from build123d import *

# Parameters (mm, degrees)
SKETCH1_R                   = 3.302
SKETCH1_R_2                 = 2.54
BOSS_EXTRUDE1_DEPTH         = 3.937
BODY_MOVE_COPY1_OUTLINE_R   = 2.54
BODY_MOVE_COPY1_DEPTH       = 3.937
BODY_MOVE_COPY1_2_OUTLINE_R = 2.54
BODY_MOVE_COPY1_2_DEPTH     = 3.937
SKETCH2_R                   = 3.302
CUT_EXTRUDE1_DEPTH          = 0.635


# Read off the part's stored shape, not the designer's step: Body-Move/Copy1
with BuildPart() as part:
    # Sketch1 → Boss-Extrude1 (new body)
    # profile 1 of 4: a face of its own
    with BuildSketch(Plane.XY):
        with BuildLine():
            Line((3.937, -3.81), (7.874, -3.81))
            ThreePointArc((7.874, -3.81), (11.684, 0), (7.874, 3.81))
            Line((7.874, 3.81), (3.937, 3.81))
            Line((3.937, 3.81), (3.937, 3.302))
            Line((3.937, 3.302), (4.92278669, 3.302))
            ThreePointArc((4.92278669, 3.302), (5.389414486, 2.994804631), (5.291688354, 2.44475))
            ThreePointArc((5.291688354, 2.44475), (4.318, 0), (5.291688354, -2.44475))
            ThreePointArc((5.291688354, -2.44475), (5.389414486, -2.994804631), (4.92278669, -3.302))
            Line((4.92278669, -3.302), (3.937, -3.302))
            Line((3.937, -3.302), (3.937, -3.81))
        make_face()
        with Locations((7.874, 0)):
            Circle(SKETCH1_R, mode=Mode.SUBTRACT)
    # profile 2 of 4: a face of its own
    with BuildSketch(Plane.XY):
        with Locations((7.874, 0)):
            Circle(SKETCH1_R)
        with Locations((7.874, 0)):
            Circle(SKETCH1_R_2, mode=Mode.SUBTRACT)
    # profile 3 of 4: a face of its own
    with BuildSketch(Plane.XY):
        with BuildLine():
            Line((-7.874, -3.81), (-3.937, -3.81))
            Line((-3.937, -3.81), (-3.937, -3.302))
            Line((-3.937, -3.302), (-4.92278669, -3.302))
            ThreePointArc((-4.92278669, -3.302), (-5.389414486, -2.994804631), (-5.291688354, -2.44475))
            ThreePointArc((-5.291688354, -2.44475), (-4.318, 0), (-5.291688354, 2.44475))
            ThreePointArc((-5.291688354, 2.44475), (-5.389414486, 2.994804631), (-4.92278669, 3.302))
            Line((-4.92278669, 3.302), (-3.937, 3.302))
            Line((-3.937, 3.302), (-3.937, 3.81))
            Line((-3.937, 3.81), (-7.874, 3.81))
            ThreePointArc((-7.874, 3.81), (-11.684, 0), (-7.874, -3.81))
        make_face()
        with Locations((-7.874, 0)):
            Circle(SKETCH1_R, mode=Mode.SUBTRACT)
    # profile 4 of 4: a face of its own
    with BuildSketch(Plane.XY):
        with Locations((-7.874, 0)):
            Circle(SKETCH1_R)
        with Locations((-7.874, 0)):
            Circle(SKETCH1_R_2, mode=Mode.SUBTRACT)
    extrude(amount=BOSS_EXTRUDE1_DEPTH)

    # Body-Move/Copy1 outline → Body-Move/Copy1 (cut)
    with BuildSketch(Plane.XY):
        with BuildLine():
            ThreePointArc((-7.874, 3.81), (-11.684, 0), (-7.874, -3.81))
            Line((-7.874, -3.81), (-3.937, -3.81))
            Line((-3.937, -3.81), (-3.937, -3.302))
            Line((-3.937, -3.302), (-4.92278669, -3.302))
            ThreePointArc((-4.92278669, -3.302), (-5.389414486, -2.994804631), (-5.291688354, -2.44475))
            ThreePointArc((-5.291688354, -2.44475), (-4.318, 0), (-5.291688354, 2.44475))
            ThreePointArc((-5.291688354, 2.44475), (-5.389414486, 2.994804631), (-4.92278669, 3.302))
            Line((-4.92278669, 3.302), (-3.937, 3.302))
            Line((-3.937, 3.302), (-3.937, 3.81))
            Line((-3.937, 3.81), (-7.874, 3.81))
        make_face()
        with Locations((-7.874, 0)):
            Circle(BODY_MOVE_COPY1_OUTLINE_R, mode=Mode.SUBTRACT)
    extrude(amount=BODY_MOVE_COPY1_DEPTH, mode=Mode.SUBTRACT)


with BuildPart() as body_2:
    # Body-Move_Copy1 2 outline → Body-Move_Copy1 2 (new body)
    with BuildSketch(Plane.XY):
        with BuildLine():
            ThreePointArc((0, 3.81), (-3.81, 0), (0, -3.81))
            Line((0, -3.81), (3.937, -3.81))
            Line((3.937, -3.81), (3.937, -3.302))
            Line((3.937, -3.302), (2.95121331, -3.302))
            ThreePointArc((2.95121331, -3.302), (2.484585514, -2.994804631), (2.582311646, -2.44475))
            ThreePointArc((2.582311646, -2.44475), (3.556, 0), (2.582311646, 2.44475))
            ThreePointArc((2.582311646, 2.44475), (2.484585514, 2.994804631), (2.95121331, 3.302))
            Line((2.95121331, 3.302), (3.937, 3.302))
            Line((3.937, 3.302), (3.937, 3.81))
            Line((3.937, 3.81), (0, 3.81))
        make_face()
        Circle(BODY_MOVE_COPY1_2_OUTLINE_R, mode=Mode.SUBTRACT)
    extrude(amount=BODY_MOVE_COPY1_2_DEPTH)


with BuildPart() as cut_extrude1_tool:
    # Sketch2 → Cut-Extrude1 (new body)
    with BuildSketch(Plane.XY):
        with Locations((7.874, 0)):
            Circle(SKETCH2_R)
        Circle(SKETCH2_R)
    extrude(amount=CUT_EXTRUDE1_DEPTH)


with BuildPart() as part_1:
    add(part.part)

    # Cut-Extrude1: cut by cut_extrude1_tool
    add(cut_extrude1_tool.part, mode=Mode.SUBTRACT)


with BuildPart() as body_2_1:
    add(body_2.part)

    # Cut-Extrude1: cut by cut_extrude1_tool
    add(cut_extrude1_tool.part, mode=Mode.SUBTRACT)


with BuildPart() as part_2:
    add(part_1.part)

    # Combine1: union body 2
    add(body_2_1.part)

    # Mirror3: part across plane


with BuildPart() as part_3:
    add(part_2.part)
    add(part_2.part.mirror(Plane.XY.offset(3.937)))


solid = part_3.part
Verification items for the finished model (mm, model axes). A direction names the side the tool comes from. Round coordinates to 2 decimals unless told otherwise and drop trailing zeros. Loops run counter-clockwise (first coordinate to the right, second up) from the corner with the lowest first, then second, coordinate; pieces in that order, holes last. Notation, with made-up numbers: (-35, 5) - (23, 5) arc R24 cw to (23, 21) - close; hole circle Ø7 at (-14.75, 52.5). An arc over 180 degrees is marked (long way). Write item = value, one per line.
Q1. Sectioned sample at A-A on y = 0. State how many separate pieces and enclosed holes the cut face has, plus the area to 3 significant figures.
Here are the results:
separate_pieces = 4
enclosed_holes = 0
area = 32.1 mm^2
Q2. Sectioned sample at B-B on x = 8.5. Record the boundary of the cut face in (y, z) (3 decimals).
Here are the results:
outline = (-3.758, 0) - (-3.242, 0) - (-3.242, 0.635) - (-2.462, 0.635) - (-2.462, 7.239) - (-3.242, 7.239) - (-3.242, 7.874) - (-3.758, 7.874) - close; (2.462, 0.635) - (3.242, 0.635) - (3.242, 0) - (3.758, 0) - (3.758, 7.874) - (3.242, 7.874) - (3.242, 7.239) - (2.462, 7.239) - close
Q3. Material ranges on L1, parallel to X at y = 0, z = 1.75; L2, parallel to X at y = -2.25, z = 4.5; L3, parallel to Y at x = 4, z = 6, recorded low to high.
Here are the results:
L1 = -3.81 to -2.54, 2.54 to 3.56, 4.32 to 5.33, 10.41 to 11.68
L2 = -3.07 to -1.18, 1.18 to 2.75, 5.12 to 6.7, 9.05 to 10.95
L3 = -3.81 to -3.3, 3.3 to 3.81
Q4. Sectioned sample at C-C on z = 4.5. Record the boundary of the cut face in (x, y), plus the area to 3 significant figures.
Here are the results:
outline = (0, -3.81) - (7.87, -3.81) arc R3.81 ccw to (7.87, 3.81) - (0, 3.81) arc R3.81 ccw to start; hole circle Ø5.08 at (0, 0); hole (2.58, -2.44) arc R0.51 ccw to (2.95, -3.3) - (4.92, -3.3) arc R0.51 ccw to (5.29, -2.44) arc R3.56 cw to (5.29, 2.44) arc R0.51 ccw to (4.92, 3.3) - (2.95, 3.3) arc R0.51 ccw to (2.58, 2.44) arc R3.56 cw to start; hole circle Ø5.08 at (7.87, 0)
area = 53.5 mm^2
Q5. Mould release check, pull along Y, two halves, no side actions. Record for faces 5 (the cylindrical face through (11.683, -0.084, 3.992)), 6 (the flat face through (4, -3.81, 4)), 7 (the flat face through (10, -2, 7.239)), 8 (the cylindrical face through (3.05, -1.26, 7.56)): +Y half, -Y half, draft (parallel to the pull), parting line (faces both ways), or undercut.
Here are the results:
face_5 = parting line
face_6 = -Y half
face_7 = undercut
face_8 = undercut
Q6. Sectioned sample at D-D on y = -2.75. Record the boundary of the cut face in (x, z) (3 decimals).
Here are the results:
outline = (-2.637, 0) - (-1.828, 0) - (-1.828, 0.635) - (1.828, 0.635) - (1.828, 0) - (2.445, 0) - (2.445, 7.874) - (1.828, 7.874) - (1.828, 7.239) - (-1.828, 7.239) - (-1.828, 7.874) - (-2.637, 7.874) - close; (5.429, 0) - (6.046, 0) - (6.046, 0.635) - (9.702, 0.635) - (9.702, 0) - (10.511, 0) - (10.511, 7.874) - (9.702, 7.874) - (9.702, 7.239) - (6.046, 7.239) - (6.046, 7.874) - (5.429, 7.874) - close
Q7. Tool access check on faces 1 (the flat face through (4, 3.81, 4)), 2 (the cylindrical face through (10.924, -1.265, 0.313)), 3 (the flat face through (4, 3.302, 4)), 4 (the cylindrical face through (10.924, -1.265, 7.561)). Record the directions out of +Z, -Z, +X, -X, +Y, -Y that give a thin tool (end or side, any length) a straight path to the whole face; none if there is none.
Here are the results:
face_1 = +Z, -Z, +X, -X, +Y
face_2 = -Z
face_3 = +Z, -Z
face_4 = +Z
Q8. Depth check by flat-ended pin: pin 1 (2 mm diameter, centred on x = -0.5, y = 0.5, fed in from +Z) (1 decimal); pin 2 (1.5 mm diameter, centred on x = -2, y = -1.5, fed in from -Z) (3 decimals). Enter the tip coordinate at first touch or a pass-through.
Here are the results:
pin_1 = through
pin_2 = 0.635
